Here's how the part is built. I have some questions about the finished solid (model axes, mm). Coordinates: 2 decimals unless noted, no trailing zeros. Loops run counter-clockwise (first coordinate to the right, second up) from the corner with the lowest first, then second, coordinate; pieces in that order, holes last. Notation, with made-up numbers: (25.25, -11.75) -> (53.25, -11.75) arc R17 ccw to (53.25, 13.25) -> close; hole circle Ø5 at (12, 31.25). An arc over 180 degrees is marked (long way). Answer as a JSON object with one key per item and string values. Group by question number.
Q1. I want a section at C-C on x = -12.5. Write out the boundary of the cut face in (y, z), then the cut area to 3 significant figures.
Q2. I want a section at A-A on z = 0.9. Write out the boundary of the cut face in (x, y).
Q3. I want a section at B-B on x = 0. Write out the boundary of the cut face in (y, z).
Q4. I want a section at D-D on y = 12.5. Write out the boundary of the cut face in (x, z).
Q5. Thinking about a two-plate mould opening in Y: for faces 1 (the flat face through (-4, -64.494, 1)), 2 (the flat face through (-4, -22, 0)), 3 (the cylindrical face through (-8.181, -3.972, 0.986)), 4 (the cylindrical face through (-25.36, 6.3, 0.99)), which applies, released by +Y, released by -Y, zero draft, split by the parting line, or undercut?
Q6. I need wall thicknesses on line 1 (Y direction, x = 0, z = 0.9); line 2 (X direction, y = -5, z = 0.5); line 3 (Y direction, x = -12, z = 0.7). Which ranges of each line are inside material? Lowest first, please.
Q7. I'm going to push a flat-ended pin straight in: pin 1 (2.5 mm diameter, centred on x = 0, y = -12.5, fed in from -Z). Where does the tip first touch, or does it pass through?
```python
from build123d import *

# Parameters (mm, degrees)
BOSS_EXTRUDE1_DEPTH = 2
SKETCH2_R           = 6
SKETCH2_R_2         = 1.5
CUT_EXTRUDE1_DEPTH  = 2
SKETCH3_R           = 3
CUT_EXTRUDE2_DEPTH  = 2


with BuildPart() as part:
    # Sketch1 → Boss-Extrude1 (new body)
    with BuildSketch(Plane.XY):
        with BuildLine():
            Line((-10.598037339, 16.961179339), (-21.950536445, 9.8676744))
            ThreePointArc((-21.950536445, 9.8676744), (-25.397665118, 6.235270644), (-26.651517775, 1.38708473))
            Line((-26.651517775, 1.38708473), (-26.651517775, -64.494263033))
            Line((-26.651517775, -64.494263033), (20, -64.494263033))
            Line((20, -64.494263033), (20, 0))
            ThreePointArc((20, 0), (9.696371827, 17.492294686), (-10.598037339, 16.961179339))
        make_face()
    extrude(amount=BOSS_EXTRUDE1_DEPTH)

    # Sketch2 → Cut-Extrude1 (cut)
    with BuildSketch(Plane.XY.offset(2)):
        Circle(SKETCH2_R)
        with Locations((12.5, 0)):
            Circle(SKETCH2_R_2)
        with Locations((0, -12.5)):
            Circle(SKETCH2_R_2)
        with Locations((-12.5, 0)):
            Circle(SKETCH2_R_2)
        with Locations((0, 12.5)):
            Circle(SKETCH2_R_2)
    extrude(amount=-CUT_EXTRUDE1_DEPTH, mode=Mode.SUBTRACT)

    # Sketch3 → Cut-Extrude2 (cut)
    with BuildSketch(Plane(origin=(0, 0, 0), x_dir=(-1, 0, 0), z_dir=(0, 0, -1))):
        with Locations((10.392304845, -6)):
            Circle(SKETCH3_R)
        with Locations((20.784609691, -12)):
            Circle(SKETCH3_R)
    extrude(amount=-CUT_EXTRUDE2_DEPTH, mode=Mode.SUBTRACT)


solid = part.part
```
Result set:
{
 "1": {"outline": "(-64.49, 0) -> (-8.13, 0) -> (-8.13, 2) -> (-64.49, 2) -> close; (-3.87, 0) -> (-1.5, 0) -> (-1.5, 2) -> (-3.87, 2) -> close; (1.5, 0) -> (15.77, 0) -> (15.77, 2) -> (1.5, 2) -> close", "area": "146 mm²"},
 "2": {"outline": "(-26.65, -64.49) -> (20, -64.49) -> (20, 0) arc R20 ccw to (-10.6, 16.96) -> (-21.95, 9.87) arc R10 ccw to (-26.65, 1.39) -> close; hole circle Ø6 at (-20.78, -12); hole circle Ø3 at (-12.5, 0); hole circle Ø6 at (-10.39, -6); hole circle Ø12 at (0, 0); hole circle Ø3 at (0, -12.5); hole circle Ø3 at (0, 12.5); hole circle Ø3 at (12.5, 0)"},
 "3": {"outline": "(-64.49, 0) -> (-14, 0) -> (-14, 2) -> (-64.49, 2) -> close; (-11, 0) -> (-6, 0) -> (-6, 2) -> (-11, 2) -> close; (6, 0) -> (11, 0) -> (11, 2) -> (6, 2) -> close; (14, 0) -> (20, 0) -> (20, 2) -> (14, 2) -> close"},
 "4": {"outline": "(-17.74, 0) -> (-1.5, 0) -> (-1.5, 2) -> (-17.74, 2) -> close; (1.5, 0) -> (15.61, 0) -> (15.61, 2) -> (1.5, 2) -> close"},
 "5": {"face 1": "released by -Y", "face 2": "zero draft", "face 3": "undercut", "face 4": "released by +Y"},
 "6": {"line 1": "y = -64.49 to -14, -11 to -6, 6 to 11, 14 to 20", "line 2": "x = -26.65 to -13.22, -7.56 to -3.32, 3.32 to 20", "line 3": "y = -64.49 to -8.53, -3.47 to -1.41, 1.41 to 16.09"},
 "7": {"pin 1": "passes through"}
}
